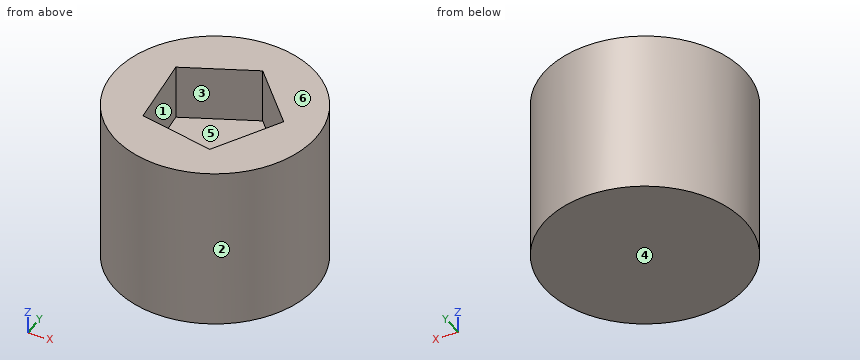
from build123d import *

# Parameters (mm, degrees)
F0_R          = 46.5572685797
F1_DEPTH      = 25.4
F2_R          = 46.5572685797
F3_DEPTH      = 25.4
F3_DEPTH_BACK = 25.4
F4_R          = 46.5572685797
F5_DEPTH      = 25.4
F8_DEPTH      = 25.4
F9_DEPTH      = 25.4


with BuildPart() as f1:
    # F0 (on Top) → F1 (new body)
    with BuildSketch(Plane.XY):
        Circle(F0_R)
    extrude(amount=F1_DEPTH)

    # F2 (on face) → F3 (join, two sides)
    with BuildSketch(Plane.XY.offset(25.4)) as f3_sk:
        Circle(F2_R)
    extrude(amount=F3_DEPTH)
    extrude(f3_sk.sketch, amount=-F3_DEPTH_BACK)

    # F4 (on face) → F5 (join)
    with BuildSketch(Plane.XY.offset(50.8)):
        Circle(F4_R)
    extrude(amount=F5_DEPTH)

    # F6 (on face) → F8 (cut)
    with BuildSketch(Plane.XY.offset(76.2)):
        Polygon((12.566284557, -27.3198056045), (29.8658746284, 3.5089625988), (5.8918410671, 29.4884637558), (-26.2245165926, 14.7159102784), (-22.0994836598, -20.3935310284), align=None)
    extrude(amount=-F8_DEPTH, mode=Mode.SUBTRACT)

    # F7 (on face) → F9 (cut)
    with BuildSketch(Plane.XY):
        Polygon((-22.0994836598, -20.3935310284), (12.566284557, -27.3198056045), (29.8658746284, 3.5089625988), (5.8918410671, 29.4884637558), (-26.2245165926, 14.7159102784), align=None)
    extrude(amount=-F9_DEPTH, mode=Mode.SUBTRACT)


solid = f1.part
The model under review builds one solid part; all positions refer to its coordinate system, in mm. Face numbers are marked on the shaded views. A direction names the side the tool comes from. Round coordinates to 2 decimals unless told otherwise and drop trailing zeros. Loops run counter-clockwise (first coordinate to the right, second up) from the corner with the lowest first, then second, coordinate; pieces in that order, holes last. Notation, with made-up numbers: M 79.25,-17 L 100.25,-17 A24 ccw 100.25,8 Z; hole C 18,65 d8. An arc over 180 degrees is marked long. Answer as CSV lines item,"result".
1. For the marked faces 5 and 6, list the 3-axis set-ups (+Z, -Z, +X, -X, +Y, -Y) from which the entire face can be reached by the end or side of a thin tool; tool diameter is ignored.
Outcome:
face 5,"+Z"
face 6,"+Z, +X, -X, +Y, -Y"
2. Draft analysis for pull direction X (two halves, no side actions). For the marked faces 1, 2, 3 and 4, state which applies: pulls with the +X half, pulls with the -X half, needs draft (parallel to the pull), parting line crosses it, or undercut.
Outcome:
face 1,"undercut"
face 2,"parting line crosses it"
face 3,"undercut"
face 4,"needs draft"
3. We need section D-D (y = -39). Give the boundary of the cut face in (x, z).
Outcome:
outline,"M -25.43,0 L 25.43,0 L 25.43,76.2 L -25.43,76.2 Z"
4. We need section C-C (y = -14). Give the boundary of the cut face in (x, z), plus the area to 3 significant figures.
Outcome:
outline,"M -44.4,0 L 44.4,0 L 44.4,76.2 L 20.04,76.2 L 20.04,50.8 L -22.85,50.8 L -22.85,76.2 L -44.4,76.2 Z"
area,"5,680 mm2"
5. We need section B-B (z = 25). Give the boundary of the cut face in (x, y).
Outcome:
outline,"C 0,0 d93.11"
6. To check wall thickness, follow L1, parallel to Y at x = -0.5, z = 33.5; L2, parallel to Z at x = -10, y = -20.5. State the ranges of each line that lie inside material, in increasing order. Write a range as [from, to].
Outcome:
L1,"y = [-46.55, 46.55]"
L2,"z = [0, 50.8]"
7. We need section A-A (x = 0). Give the boundary of the cut face in (y, z), plus the area to 4 significant figures.
Outcome:
outline,"M -46.56,0 L 46.56,0 L 46.56,76.2 L 26.78,76.2 L 26.78,50.8 L -24.81,50.8 L -24.81,76.2 L -46.56,76.2 Z"
area,"5,785 mm2"
8. Insertion check: pin 1 Ø6 at (y, z) = (18.5, 41) entering from +X; pin 2 Ø10 at (x, z) = (6, 29.5) entering from +Y; pin 3 Ø12 at (y, z) = (23, 21.5) entering from -X; pin 4 Ø2 at (x, y) = (-15, 18.5) entering from -Z. Each pin has a flat end and moves straight along its axis. Give the tip position at first contact, or say it passes through.
Outcome:
pin 1,"stops at x = 43.9"
pin 2,"stops at y = 46.55"
pin 3,"stops at x = -43.34"
pin 4,"stops at z = 0"
